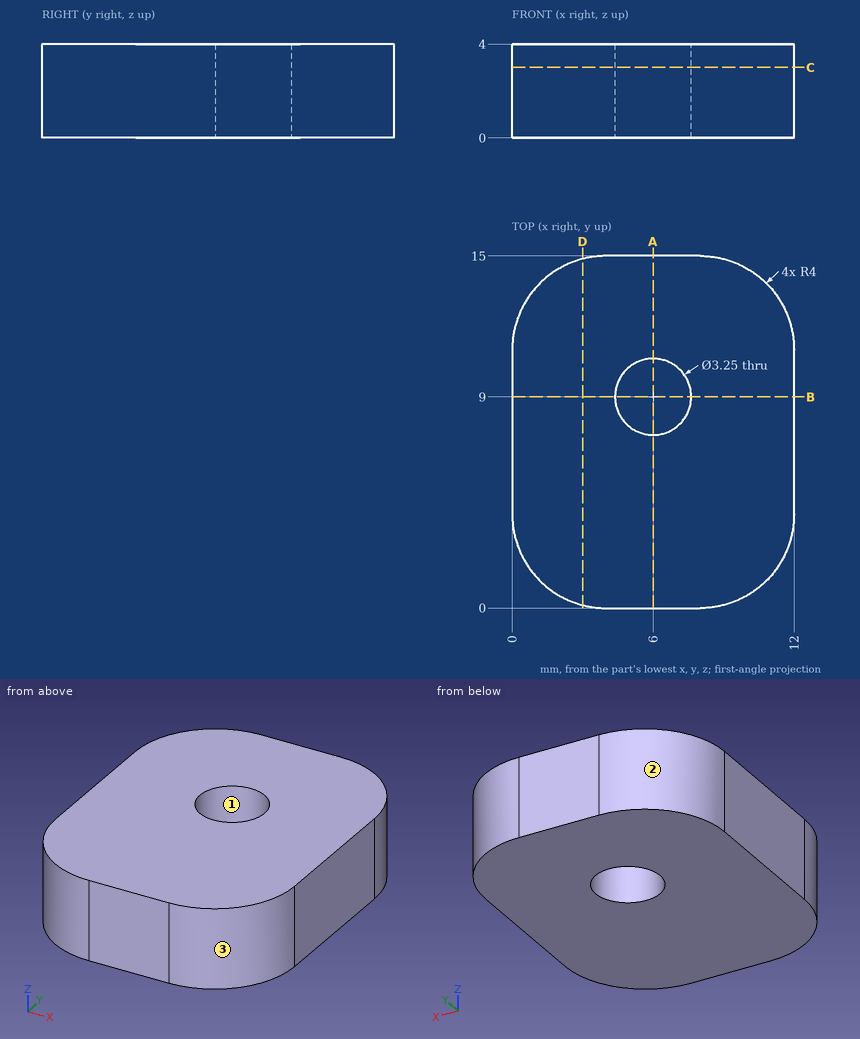
Geometry check sheet. Reference: drawing and pictorial views, mm from the part's lowest x, y, z. Coordinates: 2 decimals unless noted, no trailing zeros. Loops run counter-clockwise (first coordinate to the right, second up) from the corner with the lowest first, then second, coordinate; pieces in that order, holes last. Notation, with made-up numbers: (70, 87.25) - (103, 87.25) arc R25 cw to (103, 108.25) - close; hole circle Ø6 at (75, -16.75). An arc over 180 degrees is marked (long way). Return JSON: item names as keys, results as strings.
1. Mould release check, pull along X, two halves, no side actions. Record for the marked faces 1, 2 and 3: +X half, -X half, draft (parallel to the pull), parting line (faces both ways), or undercut.
Established:
{"face 1": "undercut", "face 2": "-X half", "face 3": "+X half"}
2. Section check B-B, the plane y = 9. Record the boundary of the cut face in (x, z) (3 decimals), then the cut area to 3 significant figures.
Established:
{"outline": "(0, 0) - (4.375, 0) - (4.375, 4) - (0, 4) - close; (7.625, 0) - (12, 0) - (12, 4) - (7.625, 4) - close", "area": "35.0 mm2"}
3. Section check D-D, the plane x = 3. Record the boundary of the cut face in (y, z), then the cut area to 3 significant figures.
Established:
{"outline": "(0.13, 0) - (14.87, 0) - (14.87, 4) - (0.13, 4) - close", "area": "59.0 mm2"}
4. Thickness scan on L1, parallel to Y at x = 6, z = 2.9 (3 decimals); L2, parallel to X at y = 8.5, z = 3.1; L3, parallel to X at y = 3.75, z = 3.1. Record the ranges inside material, lowest first.
Established:
{"L1": "y = 0 to 7.375, 10.625 to 15", "L2": "x = 0 to 4.45, 7.55 to 12", "L3": "x = 0.01 to 11.99"}
5. Section check A-A, the plane x = 6. Record the boundary of the cut face in (y, z) (3 decimals), then the cut area to 3 significant figures.
Established:
{"outline": "(0, 0) - (7.375, 0) - (7.375, 4) - (0, 4) - close; (10.625, 0) - (15, 0) - (15, 4) - (10.625, 4) - close", "area": "47.0 mm2"}
6. Section check C-C, the plane z = 3. Record the boundary of the cut face in (x, y) (3 decimals).
Established:
{"outline": "(0, 4) arc R4 ccw to (4, 0) - (8, 0) arc R4 ccw to (12, 4) - (12, 11) arc R4 ccw to (8, 15) - (4, 15) arc R4 ccw to (0, 11) - close; hole circle Ø3.25 at (6, 9)"}
